Read the model definition and answer for the solid it produces. Units are mm, in the model's axes. Face numbers are marked on the shaded views. A direction names the side the tool comes from. Coordinates: 2 decimals unless noted, no trailing zeros. Loops run counter-clockwise (first coordinate to the right, second up) from the corner with the lowest first, then second, coordinate; pieces in that order, holes last. Notation, with made-up numbers: M 66.5,-33 L 110.5,-33 A14 cw 110.5,-19 Z; hole C -23,-36 d2. An arc over 180 degrees is marked long. One line per item, written item: value. Start each with the question number.
1. For the marked faces 1, 2 and 3, determine the directions among +Z, -Z, +X, -X, +Y, -Y from which every point of the face is accessible in a straight line to the end or side of a thin tool.
2. Determine the mould class of the marked faces 4, 5 and 6 for opening direction X: +X half, -X half, draft (parallel to the pull), parting line (faces both ways), or undercut.
3. The part is cut by section A-A (z = 0). Write down the section's boundary in (x, y) (3 decimals).
4. Consider probe 1 along X at (y, z) = (1.05, 0) (3 decimals); probe 2 along Z at (x, y) = (5.75, 11.5); probe 3 along X at (y, z) = (10.25, -5.5). Determine where each line is inside the solid, lowest interval first.
5. The part is cut by section B-B (x = 0). Write down the section's boundary in (y, z) (3 decimals).
6. Flat-ended cylindrical pins translate along their axes: pin 1 (6 mm diameter, centred on x = 6, y = 5, fed in from +Z); pin 2 (1 mm diameter, centred on x = 5.5, y = 11, fed in from +Z); pin 3 (1.5 mm diameter, centred on x = 1, z = -5, fed in from +Y) (3 decimals). Find the tip coordinate at first contact, or state that the pin passes through.
7. The part is cut by section D-D (y = 11.75). Write down the section's boundary in (x, z) (3 decimals).
8. The part is cut by section C-C (z = 4). Write down the section's boundary in (x, y) (3 decimals).
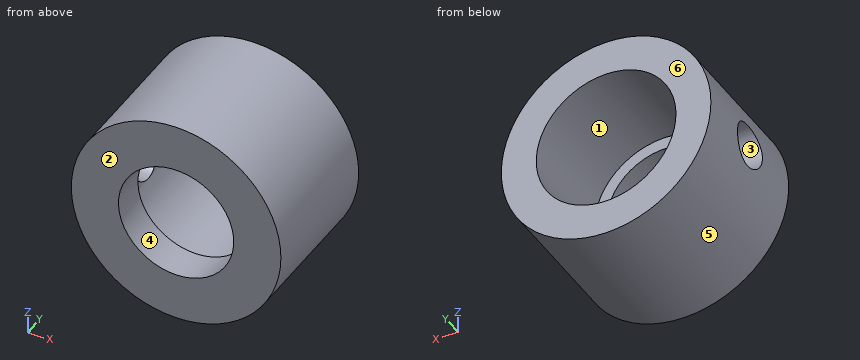
```python
from build123d import *

# Parameters (mm, degrees)
SKETCH1_R           = 9.525
BOSS_EXTRUDE1_DEPTH = 12.7
SKETCH2_R           = 6.35
CUT_EXTRUDE1_DEPTH  = 9.525
SKETCH3_R           = 2.032
CUT_EXTRUDE2_DEPTH  = 19.513272266
SKETCH4_R           = 5.23875
CUT_EXTRUDE3_DEPTH  = 19.513272438


with BuildPart() as part:
    # Sketch1 → Boss-Extrude1 (new body)
    with BuildSketch(Plane(origin=(0, 0, 0), x_dir=(1, 0, 0), z_dir=(0, 1, 0))):
        with Locations(Location((0, 0, 0), (0, 0, 270))):
            Circle(SKETCH1_R)
    extrude(amount=BOSS_EXTRUDE1_DEPTH)

    # Sketch2 → Cut-Extrude1 (cut)
    with BuildSketch(Plane(origin=(0, 12.7, 0), x_dir=(1, 0, 0), z_dir=(0, 1, 0))):
        with Locations(Location((0, 0, 0), (0, 0, 270))):
            Circle(SKETCH2_R)
    extrude(amount=-CUT_EXTRUDE1_DEPTH, mode=Mode.SUBTRACT)

    # Sketch3 → Cut-Extrude2 (cut, through all)
    with BuildSketch(Plane(origin=(0, 0, 0), x_dir=(0, 0, -1), z_dir=(1, 0, 0))):
        with Locations((0, 6.318769588)):
            Circle(SKETCH3_R)
    extrude(amount=-CUT_EXTRUDE2_DEPTH, mode=Mode.SUBTRACT)

    # Sketch4 → Cut-Extrude3 (cut, through all)
    with BuildSketch(Plane.XZ):
        with Locations(Location((0, 0, 0), (0, 0, 270))):
            Circle(SKETCH4_R)
    extrude(amount=-CUT_EXTRUDE3_DEPTH, mode=Mode.SUBTRACT)


solid = part.part
```
Answer block:
1. face 1: +Y
1. face 2: +Z, -Z, +X, -X, -Y
1. face 3: -X
2. face 4: undercut
2. face 5: parting line
2. face 6: draft
3. outline: M -9.525,0 L -5.239,0 L -5.239,3.175 L -6.35,3.175 L -6.35,4.287 L -9.525,4.287 Z; M -9.525,8.351 L -6.35,8.351 L -6.35,12.7 L -9.525,12.7 Z; M 5.239,0 L 9.525,0 L 9.525,12.7 L 6.35,12.7 L 6.35,3.175 L 5.239,3.175 Z
4. probe 1: x = -9.525 to -5.239, 5.239 to 9.525
4. probe 2: z = -7.59 to -2.69, 2.69 to 7.59
4. probe 3: x = -7.78 to -3.17, 3.17 to 7.78
5. outline: M 0,-9.525 L 12.7,-9.525 L 12.7,-6.35 L 3.175,-6.35 L 3.175,-5.239 L 0,-5.239 Z; M 0,5.239 L 3.175,5.239 L 3.175,6.35 L 12.7,6.35 L 12.7,9.525 L 0,9.525 Z
6. pin 1: stops at z = 9.04
6. pin 2: stops at z = 8.11
6. pin 3: stops at y = 3.175
7. outline: C 0,0 d19.05; hole C 0,0 d12.7
8. outline: M -8.644,0 L -3.383,0 L -3.383,3.175 L -4.932,3.175 L -4.932,12.7 L -8.644,12.7 Z; M 3.383,0 L 8.644,0 L 8.644,12.7 L 4.932,12.7 L 4.932,3.175 L 3.383,3.175 Z
